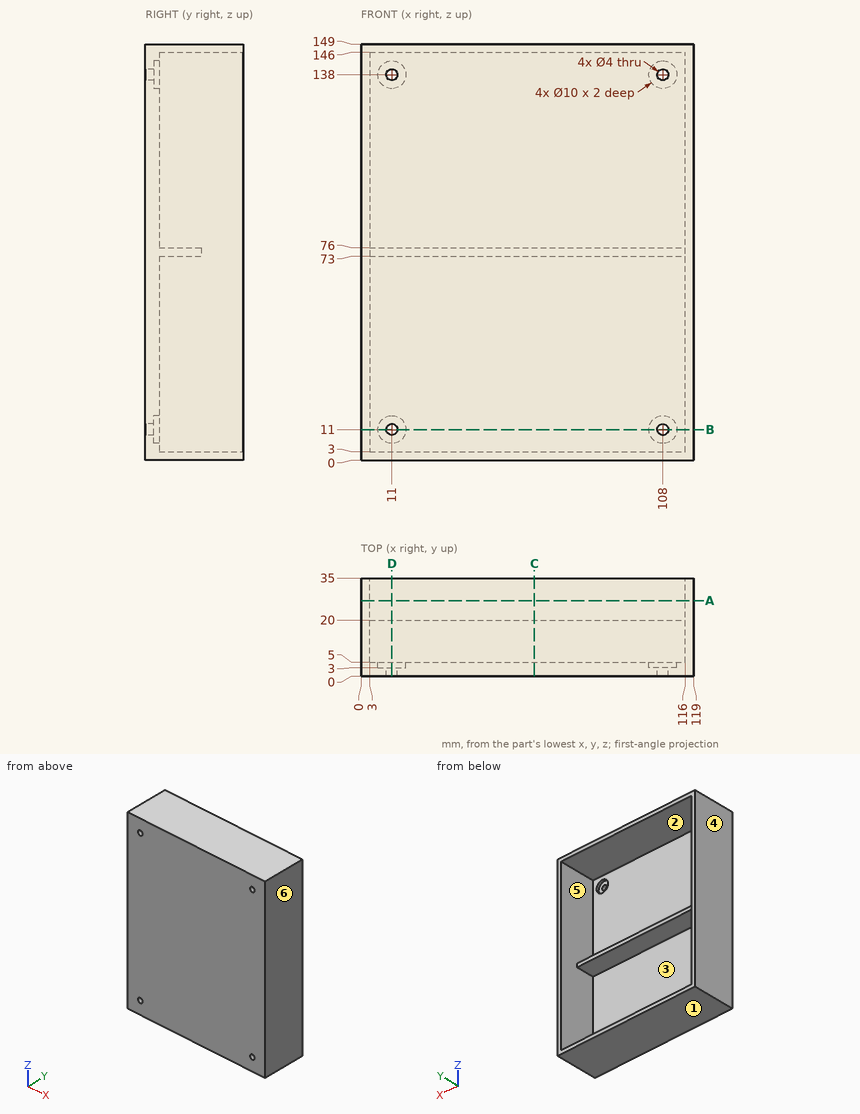
Can you work these out from the drawing? Everything is in mm from the part's minimum corner. A direction names the side the tool comes from. Give positions to 0.01 mm unless a question says otherwise; leave off trailing zeros. Order: outer loops, then holes, each group sorted by start corner. A loop starts at its lowest first (then second) coordinate and runs counter-clockwise, first axis right, second up. Notation, with made-up numbers: (-13, 50.5) -> (21, 50.5) arc R30 ccw to (21, 87.5) -> close; hole circle Ø11 at (-7.75, 65.5). An arc over 180 degrees is marked (long way). Return JSON: item names as keys, results as strings.
1. Imagine slicing it at B-B on z = 11. List the corners of the cut face in (x, y) for me, then the cut area to 3 significant figures.
Answer list:
{"outline": "(0, 0) -> (9, 0) -> (9, 3) -> (6, 3) -> (6, 5) -> (3, 5) -> (3, 35) -> (0, 35) -> close; (13, 0) -> (106, 0) -> (106, 3) -> (103, 3) -> (103, 5) -> (16, 5) -> (16, 3) -> (13, 3) -> close; (110, 0) -> (119, 0) -> (119, 35) -> (116, 35) -> (116, 5) -> (113, 5) -> (113, 3) -> (110, 3) -> close", "area": "711 mm2"}
2. Imagine slicing it at A-A on y = 27. List the corners of the cut face in (x, z) for me, then the cut area to 3 significant figures.
Answer list:
{"outline": "(0, 0) -> (119, 0) -> (119, 149) -> (0, 149) -> close; hole (3, 3) -> (116, 3) -> (116, 146) -> (3, 146) -> close", "area": "1,570 mm2"}
3. On a 3-axis mill with a long thin cutter (end or side, diameter ignored), from which of +Z, -Z, +X, -X, +Y, -Y can I reach the whole of each face in a straight line? I mean the marked faces 5 and 6. Say none if no direction works.
Answer list:
{"face 5": "+Y", "face 6": "+Z, -Z, +X, +Y, -Y"}
4. For pin 1 Ø6 at (x, z) = (11, 138) entering from +Y; pin 2 Ø0.9 at (x, z) = (67.5, 75) entering from +Y, each with a flat end and sliding along its axis, tell me the tip position at first contact or that it passes through.
Answer list:
{"pin 1": "stops at y = 3", "pin 2": "stops at y = 20"}
5. I need wall thicknesses on line 1 (X direction, y = 2.3, z = 11); line 2 (X direction, y = 4.15, z = 11); line 3 (Z direction, x = 60.5, y = 17). Which ranges of each line are inside material? Lowest first, please. Write a range as from..to.
Answer list:
{"line 1": "x = 0..9, 13..106, 110..119", "line 2": "x = 0..6, 16..103, 113..119", "line 3": "z = 0..3, 73..76, 146..149"}
6. Imagine slicing it at C-C on x = 62. List the corners of the cut face in (y, z) for me.
Answer list:
{"outline": "(0, 0) -> (35, 0) -> (35, 3) -> (5, 3) -> (5, 73) -> (20, 73) -> (20, 76) -> (5, 76) -> (5, 146) -> (35, 146) -> (35, 149) -> (0, 149) -> close"}
7. Thinking about a two-plate mould opening in Z: for the marked faces 1, 2, 3 and 4, which applies, pulls with the +Z half, pulls with the -Z half, needs draft (parallel to the pull), parting line crosses it, or undercut?
Answer list:
{"face 1": "pulls with the -Z half", "face 2": "undercut", "face 3": "undercut", "face 4": "needs draft"}
8. Imagine slicing it at D-D on x = 11. List the corners of the cut face in (y, z) for me, then the cut area to 3 significant figures.
Answer list:
{"outline": "(0, 0) -> (35, 0) -> (35, 3) -> (5, 3) -> (5, 6) -> (3, 6) -> (3, 9) -> (0, 9) -> close; (0, 13) -> (3, 13) -> (3, 16) -> (5, 16) -> (5, 73) -> (20, 73) -> (20, 76) -> (5, 76) -> (5, 133) -> (3, 133) -> (3, 136) -> (0, 136) -> close; (0, 140) -> (3, 140) -> (3, 143) -> (5, 143) -> (5, 146) -> (35, 146) -> (35, 149) -> (0, 149) -> close", "area": "906 mm2"}
